Part print with two shaded views. Sizes in mm from the minimum x, y, z corner. A direction names the side the tool comes from. Give positions to 0.01 mm unless a question says otherwise; leave off trailing zeros. Loops run counter-clockwise (first coordinate to the right, second up) from the corner with the lowest first, then second, coordinate; pieces in that order, holes last. Notation, with made-up numbers: M 81.25,-7 L 134.25,-7 A20 ccw 134.25,-2 Z; hole C 41,48.25 d3. An arc over 180 degrees is marked long. Answer in a Markdown table with one row per item.
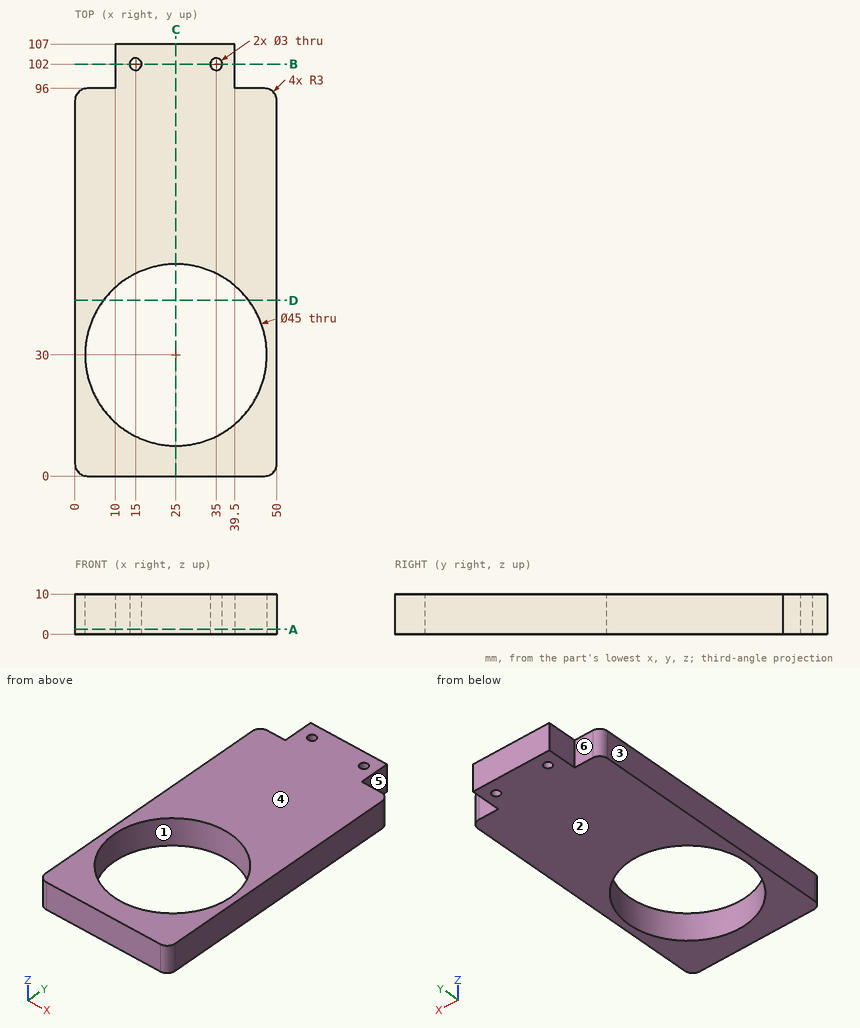
Q1. Saw through at D-D (y = 43.5). Give the cut face in (x, z).
Reported:
| item | result |
|---|---|
| outline | M 0,0 L 7,0 L 7,10 L 0,10 Z; M 43,0 L 50,0 L 50,10 L 43,10 Z |
Q2. Drop flat-ended pins along their axis: pin 1 (1.5 mm diameter, centred on x = 5.5, y = 21, fed in from -Z); pin 2 (2 mm diameter, centred on x = 6.5, z = 3.5, fed in from +Y); pin 3 (5 mm diameter, centred on y = 103.5, z = 4.5, fed in from +X). Give the stop position or say it passes through.
Reported:
| item | result |
|---|---|
| pin 1 | through |
| pin 2 | y = 96 |
| pin 3 | x = 39.5 |
Q3. Saw through at B-B (y = 102). Give the cut face in (x, z).
Reported:
| item | result |
|---|---|
| outline | M 10,0 L 13.5,0 L 13.5,10 L 10,10 Z; M 16.5,0 L 33.5,0 L 33.5,10 L 16.5,10 Z; M 36.5,0 L 39.5,0 L 39.5,10 L 36.5,10 Z |
Q4. Mould opens along X. For the marked faces 1, 2 and 3 say: released by +X, released by -X, zero draft, split by the parting line, or undercut.
Reported:
| item | result |
|---|---|
| face 1 | undercut |
| face 2 | zero draft |
| face 3 | released by -X |
Q5. 3-axis set-ups, long thin cutter, end or side, ignore diameter. For the marked faces 4, 5 and 6: which of +Z, -Z, +X, -X, +Y, -Y reach the whole face in a straight line?
Reported:
| item | result |
|---|---|
| face 4 | +Z, +X, -X, +Y, -Y |
| face 5 | +Z, -Z, +X, +Y |
| face 6 | +Z, -Z, -X, +Y |
Q6. Probe probe 1 along Y at (x, z) = (25, 6.25); probe 2 along Y at (x, z) = (15, 4); probe 3 along X at (y, z) = (36, 7). List the from-to ranges inside material, lowest first.
Reported:
| item | result |
|---|---|
| probe 1 | 0 to 7.5, 52.5 to 107 |
| probe 2 | 0 to 9.84, 50.16 to 100.5, 103.5 to 107 |
| probe 3 | 0 to 3.31, 46.69 to 50 |
Q7. Saw through at C-C (x = 25). Give the cut face in (y, z).
Reported:
| item | result |
|---|---|
| outline | M 0,0 L 7.5,0 L 7.5,10 L 0,10 Z; M 52.5,0 L 107,0 L 107,10 L 52.5,10 Z |
Q8. Saw through at A-A (z = 1.25). Give the cut face in (x, y), and give its area (3 significant figures).
Reported:
| item | result |
|---|---|
| outline | M 0,3 A3 ccw 3,0 L 47,0 A3 ccw 50,3 L 50,93 A3 ccw 47,96 L 39.5,96 L 39.5,107 L 10,107 L 10,96 L 3,96 A3 ccw 0,93 Z; hole C 25,30 d45; hole C 15,102 d3; hole C 35,102 d3 |
| area | 3,510 mm² |
